CAD build for the part. Positions are in the model's coordinates, mm. Give positions to 0.01 mm unless a question says otherwise; leave off trailing zeros. Order: outer loops, then holes, each group sorted by start corner. A loop starts at its lowest first (then second) coordinate and runs counter-clockwise, first axis right, second up.
from build123d import *

# Parameters (mm, degrees)
SKETCH1_R               = 1.984375
BOSS_EXTRUDE1_DEPTH     = 169.87265999999997
CUT_EXTRUDE1_DEPTH      = 23.05812
CUT_EXTRUDE2_START      = -169.87266
CUT_EXTRUDE2_DEPTH      = 23.05812
FILLET1_R               = 7.62
CUT_EXTRUDE3_DEPTH      = 198.3909425992125
CUT_EXTRUDE3_DEPTH_BACK = 198.3909425992125
SKETCH6_R               = 2.100000000000005
SKETCH6_R_2             = 2.0999999999999983
CUT_EXTRUDE4_DEPTH      = 198.3909425992125
CUT_EXTRUDE4_DEPTH_BACK = 198.3909425992125
SKETCH7_W               = 96.26632678346117
SKETCH7_H               = 79.91099312056471
SKETCH7_H_2             = 50.31480687943524
CUT_EXTRUDE5_DEPTH      = 109.06635501646407
CUT_EXTRUDE5_DEPTH_BACK = 109.06635501646407


with BuildPart() as part:
    # Sketch1 → Boss-Extrude1 (new body)
    with BuildSketch(Plane(origin=(0, 0, 0), x_dir=(1, 0, 0), z_dir=(0, 1, 0))):
        with BuildLine():
            Line((-9.955287346489113, -3.6074515728352274), (-6.769721367669625, -3.607451572835229))
            Line((-6.769721367669625, -3.607451572835229), (8.985913588520251, -3.607451572835254))
            Line((8.985913588520251, -3.607451572835254), (12.171479567676489, -3.6074515728352536))
            add(Edge.make_bspline(
                [(10.60289964969583, -20.752451572835255), (11.099968974105767, -15.73020157118813), (11.63056361676113, -10.016003165571346), (12.11399787104698, -4.2968169522780775), (12.171479567676489, -3.6074515728352536)],
                knots=[0.38496962590391054, 0.38496962590391054, 0.38496962590391054, 0.38496962590391054, 0.4581086713676085, 0.468131593311824, 0.468131593311824, 0.468131593311824, 0.468131593311824], degree=3))
            add(Edge.make_bspline(
                [(1.1080961105936413, -99.87377835629641), (4.527344743513008, -73.5317641629186), (7.98655990047842, -47.187219651543), (10.60289964969583, -20.752451572835255)],
                knots=[0, 0, 0, 0, 0.38496962590391054, 0.38496962590391054, 0.38496962590391054, 0.38496962590391054], degree=3))
            add(Edge.make_bspline(
                [(1.1080961105936413, -99.87377835629641), (-2.311152522316452, -73.53176416292023), (-5.77036767929202, -47.18721965154205), (-8.386707428509173, -20.752451572835213)],
                knots=[0, 0, 0, 0, 0.3849696259039116, 0.3849696259039116, 0.3849696259039116, 0.3849696259039116], degree=3))
            add(Edge.make_bspline(
                [(-8.386707428509173, -20.752451572835213), (-8.88377675291906, -15.730201571188243), (-9.414371395575625, -10.016003165551679), (-9.897805649859514, -4.29681695227938), (-9.955287346489113, -3.6074515728352274)],
                knots=[0.3849696259039116, 0.3849696259039116, 0.3849696259039116, 0.3849696259039116, 0.4581086713676079, 0.46813159331185, 0.46813159331185, 0.46813159331185, 0.46813159331185], degree=3))
        make_face()
        with Locations(Location((1.10810856874065, -11.326456678177, 0), (0, 0, 270))):
            Circle(SKETCH1_R, mode=Mode.SUBTRACT)
    extrude(amount=BOSS_EXTRUDE1_DEPTH)

    # Sketch2 → Cut-Extrude1 (cut)
    with BuildSketch(Plane(origin=(0, 169.87265999999997, 0), x_dir=(1, 0, 0), z_dir=(0, 1, 0))):
        Polygon((-9.955287346489113, -3.6074515728352274), (25.808519749497883, -3.6074515728352274), (25.808519749497883, -26.312456678177), (-9.95528734648911, -26.312456678177), align=None)
    extrude(amount=-CUT_EXTRUDE1_DEPTH, mode=Mode.SUBTRACT)

    # Sketch2<2> → Cut-Extrude2 (cut)
    with BuildSketch(Plane(origin=(0, 169.87265999999997, 0), x_dir=(1, 0, 0), z_dir=(0, 1, 0)).offset(CUT_EXTRUDE2_START)):
        Polygon((-9.955287346489113, -3.6074515728352274), (25.808519749497883, -3.6074515728352274), (25.808519749497883, -26.312456678177), (-9.95528734648911, -26.312456678177), align=None)
    extrude(amount=CUT_EXTRUDE2_DEPTH, mode=Mode.SUBTRACT)

    # Fillet1
    fillet1_edges = [part.edges().sort_by_distance(p)[0] for p in [
        (-7.8241553741226255, 11.529059999999971, 26.312456678177),
        (10.04034759530939, 11.529059999999971, 26.312456678177),
        (-9.955287346489113, 84.93632999999997, 3.6074515728352274),
        (12.171479567676489, 84.93632999999997, 3.6074515728352536),
        (-7.8241553741226255, 158.34359999999998, 26.312456678177),
        (10.04034759530939, 158.34359999999998, 26.312456678177),
    ]]
    fillet(fillet1_edges, radius=FILLET1_R)

    # Sketch6 → Cut-Extrude3 (cut, two sides: drawn at the far end of the back side and taken through both)
    with BuildSketch(Plane.XZ.offset(-CUT_EXTRUDE3_DEPTH_BACK)):
        with Locations(Location((1.1080961105936413, 71.9337783562964, 0), (0, 0, 270))):
            Circle(SKETCH6_R)
        with Locations(Location((1.1080961105935272, 34.76055213743882, 0), (0, 0, 270))):
            Circle(SKETCH6_R_2)
    extrude(amount=CUT_EXTRUDE3_DEPTH + CUT_EXTRUDE3_DEPTH_BACK, mode=Mode.SUBTRACT)

    # Sketch7 → Cut-Extrude4 (cut, two sides: drawn at the far end of the back side and taken through both)
    with BuildSketch(Plane(origin=(0, 0, 0), x_dir=(0, 0, -1), z_dir=(1, 0, 0)).offset(-CUT_EXTRUDE4_DEPTH_BACK)):
        with Locations((-51.740614964565815, 39.955496560282356)):
            Rectangle(SKETCH7_W, SKETCH7_H)
        with Locations((-51.740614964565815, 144.71525656028234)):
            Rectangle(SKETCH7_W, SKETCH7_H_2)
    extrude(amount=CUT_EXTRUDE4_DEPTH + CUT_EXTRUDE4_DEPTH_BACK, mode=Mode.SUBTRACT)

    # Sketch8 → Cut-Extrude5 (cut, two sides: drawn at the far end of the back side and taken through both)
    with BuildSketch(Plane.XZ.offset(-79.91099312056471).offset(-CUT_EXTRUDE5_DEPTH_BACK)):
        Polygon((-35.738182727497644, 136.6065064389988), (32.4461710118659, 136.6065064389988), (32.446171011865914, 16.307451572835227), (-35.73818272749763, 16.307451572835227), align=None)
    extrude(amount=CUT_EXTRUDE5_DEPTH + CUT_EXTRUDE5_DEPTH_BACK, mode=Mode.SUBTRACT)


solid = part.part
1. Saw through at A-A on x = 2. Give the cut face in (y, z), plus the area to 3 significant figures.
2. Pin check, flat tips, straight feed: P1, Ø3, axis at y = 102.5, z = 6.5, coming from the +X side; P2, Ø2, axis at y = 97, z = 8, coming from the -X side; P3, Ø3.5, axis at x = 1.11, z = 11.33, coming from the +Y side. Stop position of each tip, or through.
3. Saw through at B-B on x = -0.5. Give the cut face in (y, z), plus the area to 3 significant figures.
4. Wall check: line 1 (Z direction, x = 0.75, y = 95); line 2 (X direction, y = 92, z = 12.5); line 3 (X direction, y = 96, z = 13). Give the ranges that are in metal, low to high.
5. Mould opens along X. For faces 1 (the cylindrical face through (1.7, 99.46, 13.22)), 2 (the flat face through (1, 100, 16.307)) say: released by +X, released by -X, zero draft, split by the parting line, or undercut.
Reported:
1. outline: (79.91, 3.61) - (119.56, 3.61) - (119.56, 9.55) - (79.91, 9.55) - close; (79.91, 13.1) - (119.56, 13.1) - (119.56, 16.31) - (79.91, 16.31) - close
1. area: 363 mm2
2. P1: stops at x = 10.76
2. P2: stops at x = -8.93
2. P3: passes through
3. outline: (79.91, 3.61) - (119.56, 3.61) - (119.56, 10.16) - (79.91, 10.16) - close; (79.91, 12.49) - (119.56, 12.49) - (119.56, 16.31) - (79.91, 16.31) - close
3. area: 411 mm2
4. line 1: z = 3.61 to 9.37, 13.28 to 16.31
4. line 2: x = -9.17 to -0.49, 2.71 to 11.39
4. line 3: x = -9.13 to 0.04, 2.17 to 11.34
5. face 1: undercut
5. face 2: zero draft
